from build123d import *

# Parameters (mm, degrees)
SKETCH1_W           = 80
SKETCH1_H           = 45
BOSS_EXTRUDE1_DEPTH = 10
SKETCH2_W           = 110
SKETCH2_H           = 12
CUT_EXTRUDE1_DEPTH  = 7.8
SKETCH4_R           = 2
CUT_EXTRUDE3_DEPTH  = 11
SKETCH5_R           = 3.5
CUT_EXTRUDE4_DEPTH  = 3


with BuildPart() as part:
    # Sketch1 → Boss-Extrude1 (new body)
    with BuildSketch(Plane.XY):
        with Locations((40, 22.5)):
            Rectangle(SKETCH1_W, SKETCH1_H)
    extrude(amount=BOSS_EXTRUDE1_DEPTH)

    # Sketch2 → Cut-Extrude1 (cut)
    with BuildSketch(Plane(origin=(0, 0, 0), x_dir=(-1, 0, 0), z_dir=(0, 0, -1))):
        with Locations((-25, 22.5)):
            Rectangle(SKETCH2_W, SKETCH2_H)
    extrude(amount=-CUT_EXTRUDE1_DEPTH, mode=Mode.SUBTRACT)

    # Sketch4 → Cut-Extrude3 (cut, through all)
    with BuildSketch(Plane.XY.offset(10)):
        with Locations((10, 37.5)):
            Circle(SKETCH4_R)
        with Locations((70, 37.5)):
            Circle(SKETCH4_R)
        with Locations((70, 7.5)):
            Circle(SKETCH4_R)
        with Locations((10, 7.5)):
            Circle(SKETCH4_R)
    extrude(amount=-CUT_EXTRUDE3_DEPTH, mode=Mode.SUBTRACT)

    # Sketch5 → Cut-Extrude4 (cut)
    with BuildSketch(Plane.XY.offset(10)):
        with Locations((10, 37.5)):
            Circle(SKETCH5_R)
        with Locations((70, 37.5)):
            Circle(SKETCH5_R)
        with Locations((70, 7.5)):
            Circle(SKETCH5_R)
        with Locations((10, 7.5)):
            Circle(SKETCH5_R)
    extrude(amount=-CUT_EXTRUDE4_DEPTH, mode=Mode.SUBTRACT)


solid = part.part
Check sheet for the modelled part. Datum: model origin and axes. Units: mm. A direction names the side the tool comes from. Round coordinates to 2 decimals unless told otherwise and drop trailing zeros. Loops run counter-clockwise (first coordinate to the right, second up) from the corner with the lowest first, then second, coordinate; pieces in that order, holes last. Notation, with made-up numbers: M -4.75,2.5 L 24.25,2.5 A24 cw 24.25,34.5 Z; hole C 48.5,-5 d8. An arc over 180 degrees is marked long. One line per question, with ' | ' between items. Start each with the question number.
Item 1: Section check A-A (z = 3.75). Record the boundary of the cut face in (x, y), and give its area (3 significant figures).
Item 2: Release check for a two-part mould opening along X. For faces 1 (the face through (80, 22, 8)), 2 (the face through (39, 0, 5)), 3 (the face through (7.2, 5.4, 8.5)) record: released by +X, released by -X, zero draft, split by the parting line, or undercut.
Item 3: Section check C-C (x = 10). Record the boundary of the cut face in (y, z).
Item 4: Section check B-B (y = 37.5). Record the boundary of the cut face in (x, z).
Item 5: Section check D-D (x = 58.5). Record the boundary of the cut face in (y, z).
Item 6: Gauge pin test, flat ends, axial feed: pin 1 Ø2 at (y, z) = (6, 5) entering from -X; pin 2 Ø2 at (x, y) = (71, 6) entering from +Z; pin 3 Ø3.5 at (x, y) = (21.5, 20) entering from -Z. Record the tip position at first contact, or that the pin passes through.
Item 7: Scan lines: probe 1 along Y at (x, z) = (70, 3); probe 2 along Y at (x, z) = (70, 7.75); probe 3 along Y at (x, z) = (36, 1.5). Record each from-to range of solid material in increasing order.
Item 8: Set-up check for faces 4 (the face through (41, 23, 7.8)), 5 (the face through (70.923, 35.726, 3.549)), 6 (the face through (12, 6, 7)): record each of +Z, -Z, +X, -X, +Y, -Y from which the full face is reachable in a straight line by a thin tool's end or side.
Worked out:
1) outline: M 0,0 L 80,0 L 80,16.5 L 0,16.5 Z; M 0,28.5 L 80,28.5 L 80,45 L 0,45 Z; hole C 10,7.5 d4; hole C 10,37.5 d4; hole C 70,7.5 d4; hole C 70,37.5 d4 | area: 2,590 mm^2
2) face 1: released by +X | face 2: zero draft | face 3: undercut
3) outline: M 0,0 L 5.5,0 L 5.5,7 L 4,7 L 4,10 L 0,10 Z; M 9.5,0 L 16.5,0 L 16.5,7.8 L 28.5,7.8 L 28.5,0 L 35.5,0 L 35.5,7 L 34,7 L 34,10 L 11,10 L 11,7 L 9.5,7 Z; M 39.5,0 L 45,0 L 45,10 L 41,10 L 41,7 L 39.5,7 Z
4) outline: M 0,0 L 8,0 L 8,7 L 6.5,7 L 6.5,10 L 0,10 Z; M 12,0 L 68,0 L 68,7 L 66.5,7 L 66.5,10 L 13.5,10 L 13.5,7 L 12,7 Z; M 72,0 L 80,0 L 80,10 L 73.5,10 L 73.5,7 L 72,7 Z
5) outline: M 0,0 L 16.5,0 L 16.5,7.8 L 28.5,7.8 L 28.5,0 L 45,0 L 45,10 L 0,10 Z
6) pin 1: x = 0 | pin 2: z = 7 | pin 3: z = 7.8
7) probe 1: 0 to 5.5, 9.5 to 16.5, 28.5 to 35.5, 39.5 to 45 | probe 2: 0 to 4, 11 to 16.5, 28.5 to 34, 41 to 45 | probe 3: 0 to 16.5, 28.5 to 45
8) face 4: -Z, +X, -X | face 5: +Z, -Z | face 6: +Z
